For this review, take the finished solid that the model builds, in its own axes (mm). Coordinates: 2 decimals unless noted, no trailing zeros. Loops run counter-clockwise (first coordinate to the right, second up) from the corner with the lowest first, then second, coordinate; pieces in that order, holes last. Notation, with made-up numbers: M 33,27 L 64,27 A15 cw 64,42 Z; hole C 42.25,40.25 d3. An arc over 180 degrees is marked long. Answer as a JSON object with one key per item and string values. Group by question number.
Item 1: Add section A-A (x = 6.5). State the section outline as (y, z) points.
Item 2: Add section C-C (z = 15). State the section outline as (x, y) points.
Item 3: Wall thickness on L1, parallel to Y at x = 0, z = 15; L2, parallel to Z at x = 15, y = -32.5; L3, parallel to Y at x = 13, z = 4.5: over which ranges is each line inside the solid? List them lowest first. Write a range as from..to.
Item 4: Add section D-D (y = -26.5). State the section outline as (x, z) points, then the cut area to 3 significant figures.
Item 5: Insertion check: pin 1 (5 mm diameter, centred on x = 10.5, y = 13.5, fed in from -Z); pin 2 (4 mm diameter, centred on x = 0, y = 27, fed in from +Z). Each pin has a flat end and moves straight along its axis. Give the tip position at first contact, or say it passes through.
Item 6: Add section B-B (y = 0). State the section outline as (x, z) points, then the cut area to 3 significant figures.
from build123d import *

# Parameters (mm, degrees)
F0_W     = 43.5707718134
F0_H     = 77.7630805969
F0_R     = 14.0639610487
F1_DEPTH = 25.4
F2_W     = 33.0200046301
F2_H     = 38.6861525476
F3_DEPTH = 25.4
F3_TAPER = 50
F4_R     = 14.0639610487
F5_DEPTH = 25.4


with BuildPart() as f1:
    # F0 (on Top) → F1 (new body)
    with BuildSketch(Plane.XY):
        Rectangle(F0_W, F0_H)
        Circle(F0_R, mode=Mode.SUBTRACT)
    extrude(amount=F1_DEPTH)

    # F2 (on face) → F3 (join)
    with BuildSketch(Plane.XY.offset(25.4)):
        Rectangle(F2_W, F2_H)
    extrude(amount=F3_DEPTH, taper=F3_TAPER)

    # F4 (on face) → F5 (cut)
    with BuildSketch(Plane(origin=(0, 0, 25.4), x_dir=(1, 0, 0), z_dir=(0, 0, -1))):
        Circle(F4_R)
    extrude(amount=-F5_DEPTH, mode=Mode.SUBTRACT)


solid = f1.part
From the geometry:
{
 "1": {"outline": "M -38.88,0 L -12.47,0 L -12.47,31.17 L -19.34,25.4 L -38.88,25.4 Z; M 12.47,0 L 38.88,0 L 38.88,25.4 L 19.34,25.4 L 12.47,31.17 Z"},
 "2": {"outline": "M -21.79,-38.88 L 21.79,-38.88 L 21.79,38.88 L -21.79,38.88 Z; hole C 0,0 d28.13"},
 "3": {"L1": "y = -38.88..-14.06, 14.06..38.88", "L2": "z = 0..25.4", "L3": "y = -38.88..-5.37, 5.37..38.88"},
 "4": {"outline": "M -21.79,0 L 21.79,0 L 21.79,25.4 L -21.79,25.4 Z", "area": "1,110 mm²"},
 "5": {"pin 1": "stops at z = 0", "pin 2": "stops at z = 25.4"},
 "6": {"outline": "M -21.79,0 L -14.06,0 L -14.06,27.45 L -16.51,25.4 L -21.79,25.4 Z; M 14.06,0 L 21.79,0 L 21.79,25.4 L 16.51,25.4 L 14.06,27.45 Z", "area": "397 mm²"}
}
